Design review of the part built by this model. Coordinates are the model's own, in mm. Face numbers are marked on the shaded views. A direction names the side the tool comes from. Round coordinates to 2 decimals unless told otherwise and drop trailing zeros. Order: outer loops, then holes, each group sorted by start corner. A loop starts at its lowest first (then second) coordinate and runs counter-clockwise, first axis right, second up. Notation, with made-up numbers: M 75.25,-19.5 L 93.25,-19.5 A32 ccw 93.25,14.5 Z; hole C -38,-6.75 d7. An arc over 180 degrees is marked long. Write item = value, one per line. Start each with the question number.
Autodesk Inventor part; units mm, degrees
ref_plane "YZ Plane" through (0, 0, 0) normal (1, 0, 0) x (0, 1, 0)
ref_plane "XZ Plane" through (0, 0, 0) normal (0, 1, 0) x (-1, 0, 0)
ref_plane "XY Plane" through (0, 0, 0) normal (0, 0, 1) x (1, 0, 0)
sketch "Sketch1" plane through (0, 0, 0) normal (0, 0, 1) x (1, 0, 0)
  circle A0 centre (0, 0) radius 20
  dimension "d0" = 40
extrude "Extrusion1" add sketch "Sketch1" along normal blind 24
sketch "Sketch2" plane through (0, 0, 24) normal (0, 0, 1) x (1, 0, 0)
  arc A0 (-9.5263, 5.5) -> (-9.5263, -5.5) centre (0, 0) ccw
  line L0 (-9.5263, 5.5) -> (-17.3205, 10)
  circle A1 centre (0, 0) radius 20
  line L1 (0, 0) -> (20, 0) construction
  line L2 (-9.5263, -5.5) -> (-17.3205, -10)
  line L3 (0, 0) -> (20, 0) construction
  line L4 (0, 0) -> (0, 20) construction
  arc A2 (9.5263, -5.5) -> (9.5263, 5.5) centre (0, 0) ccw
  line L5 (9.5263, 5.5) -> (17.3205, 10)
  line L6 (9.5263, -5.5) -> (17.3205, -10)
  dimension "d3" = 22
  dimension "d4" = 150
  dimension "d5" = 150
extrude "Extrusion2" add sketch "Sketch2" along normal blind 17 contours A0 L2 A1 L0 | A1 L6 A2 L5
sketch "Sketch3" plane through (0, 0, 24) normal (0, 0, 1) x (1, 0, 0)
  circle A0 centre (0, 0) radius 11
  dimension "d8" = 22
extrude "Extrusion3" cut sketch "Sketch3" against normal through all
properties part number "22MM JAW"
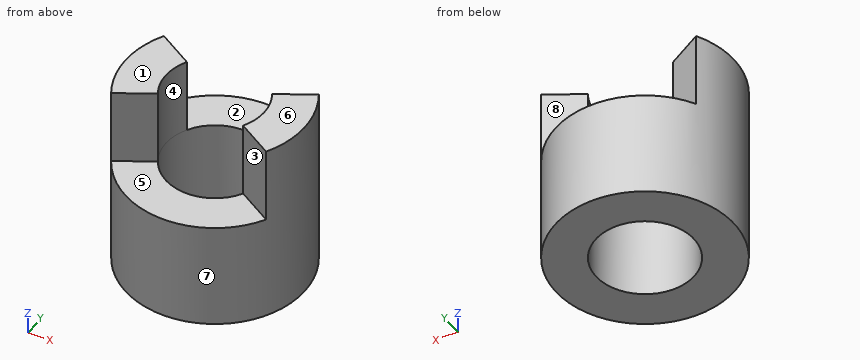
(1) Consider section A-A, the plane z = 33. Write out the cut boundary in (x, y).
(2) Consider section D-D, the plane x = 12. Write out the cut boundary in (y, z), then the cut area to 3 significant figures.
(3) Consider section B-B, the plane x = 0. Write out the cut boundary in (y, z), then the cut area to 3 significant figures.
(4) Insertion check: pin 1 (3 mm diameter, centred on x = 9.5, z = 35.5, fed in from -Y); pin 2 (1.5 mm diameter, centred on x = -9.5, z = 19, fed in from +Y); pin 3 (16 mm diameter, centred on x = 3, y = -11, fed in from +Z). Each pin has a flat end and moves straight along its axis. Give the tip position at first contact, or say it passes through.
(5) For the marked faces 1, 2, 3 and 4, list the 3-axis set-ups (+Z, -Z, +X, -X, +Y, -Y) from which the entire face can be reached by the end or side of a thin tool; tool diameter is ignored.
(6) Draft analysis for pull direction X (two halves, no side actions). For the marked faces 5, 6, 7 and 8, state which applies: pulls with the +X half, pulls with the -X half, needs draft (parallel to the pull), parting line crosses it, or undercut.
(7) For line 1 along Y through (x, z) = (0, 15); line 2 along Z through (x, y) = (-11, -16.5), list the stretches that pass through material, from the lowest coordinate up. Write a range as [from, to].
(8) Consider section C-C, the plane y = -8.5. Write out the cut boundary in (x, z).
Completed:
q1.outline = M -17.32,-10 L -9.53,-5.5 A11 cw -9.53,5.5 L -17.32,10 A20 ccw Z; M 9.53,-5.5 L 17.32,-10 A20 ccw 17.32,10 L 9.53,5.5 A11 cw Z
q2.outline = M -16,0 L 16,0 L 16,24 L 6.93,24 L 6.93,41 L -6.93,41 L -6.93,24 L -16,24 Z
q2.area = 1,000 mm2
q3.outline = M -20,0 L -11,0 L -11,24 L -20,24 Z; M 11,0 L 20,0 L 20,24 L 11,24 Z
q3.area = 432 mm2
q4.pin_1 = -6.35
q4.pin_2 = 17.98
q4.pin_3 = 24
q5.face_1 = +Z, +X, -X, +Y, -Y
q5.face_2 = +Z, +Y
q5.face_3 = +Z, -Y
q5.face_4 = +Z, -Z
q6.face_5 = undercut
q6.face_6 = needs draft
q6.face_7 = parting line crosses it
q6.face_8 = undercut
q7.line_1 = [-20, -11], [11, 20]
q7.line_2 = [0, 24]
q8.outline = M -18.1,0 L -6.98,0 L -6.98,24 L -14.72,24 L -14.72,41 L -18.1,41 Z; M 6.98,0 L 18.1,0 L 18.1,41 L 14.72,41 L 14.72,24 L 6.98,24 Z
